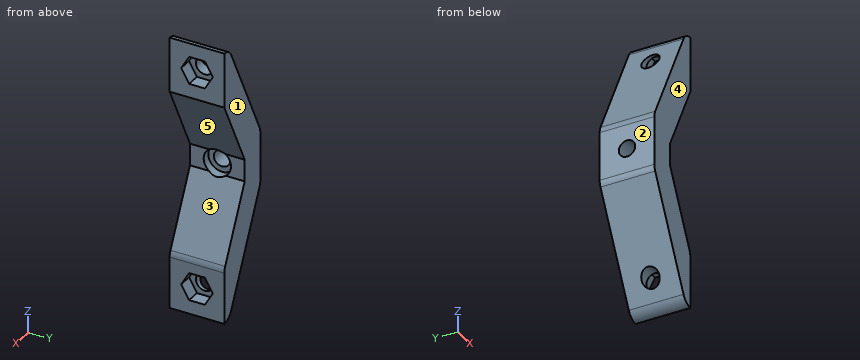
Autodesk Inventor part; units mm, degrees
ref_plane "YZ Plane" through (0, 0, 0) normal (1, 0, 0) x (0, 1, 0)
ref_plane "XZ Plane" through (0, 0, 0) normal (0, 1, 0) x (-1, 0, 0)
ref_plane "XY Plane" through (0, 0, 0) normal (0, 0, 1) x (1, 0, 0)
sketch "Sketch1" plane through (0, 0, 0) normal (0, 1, 0) x (-1, 0, 0)
  line L0 (0, 0) -> (-20, 0)
  line L1 (-20, 0) -> (-20, -40)
  line L2 (-20, -40) -> (0, 0)
  line L3 (-21.5, -50) -> (-18.5, -50)
  line L4 (-18.5, -50) -> (-18.5, -30)
  line L5 (-18.5, -30) -> (-21.5, -30)
  line L6 (-21.5, -30) -> (-21.5, -50)
  line L7 (-21.5, -50) -> (-18.5, -30) construction
  line L8 (-18.5, -50) -> (-21.5, -30) construction
  line L9 (1.5, 10) -> (-1.5, 10)
  line L10 (-1.5, 10) -> (-1.5, -10)
  line L11 (-1.5, -10) -> (1.5, -10)
  line L12 (1.5, -10) -> (1.5, 10)
  line L13 (1.5, 10) -> (-1.5, -10) construction
  line L14 (-1.5, 10) -> (1.5, -10) construction
  line L15 (-1.5, 10) -> (-21.5, -30)
  line L16 (1.5, -10) -> (-18.5, -50)
  line L17 (1.5, -10) -> (1.5, 10)
  line L18 (1.5, -10) -> (1.5, 10)
  line L19 (1.5, 10) -> (-8.5, 10)
  line L20 (-8.5, 10) -> (-8.5, -10)
  line L21 (-8.5, -10) -> (1.5, -10)
  line L22 (1.5, -10) -> (1.5, 10)
  line L23 (0, 0) -> (10, 0)
  line L24 (0, 0) -> (10, 0) construction
  line L25 (-20, 40) -> (0, 0)
  line L26 (-21.5, 50) -> (-18.5, 50)
  line L27 (-18.5, 50) -> (-18.5, 30)
  line L28 (-18.5, 30) -> (-21.5, 30)
  line L29 (-21.5, 30) -> (-21.5, 50)
  line L30 (-1.5, -10) -> (-1.5, 10)
  line L31 (-1.5, 10) -> (1.5, 10)
  line L32 (-1.5, -10) -> (-21.5, 30)
  line L33 (1.5, 10) -> (-18.5, 50)
  line L34 (1.5, 10) -> (1.5, -10)
  point P0 (-7.3579, -1.7157)
  point P1 (-11.5, -10)
  point P2 (-11.5, -10)
  point P3 (-8.5, -4)
  point P4 (-8.5, 4)
  dimension "d0" = 20
  dimension "d1" = 40
  dimension "d2" = 3
  dimension "d3" = 20
  dimension "d4" = 3
  dimension "d5" = 20
  dimension "d31" = 10
  dimension "d32" = 20
  dimension "d42" = 10
  dimension "d43" = 0
extrude "Extrusion1" add sketch "Sketch1" along normal blind 20 contours L2 L10 L0 | L23 L12 L11 L10 L2 | L25 L10 L9 L12 L23 | L0 L10 L25 | L10 L2 L32 L0 | L0 L15 L25 L10 | L10 L32 L2 | L25 L15 L10 | L15 L20 L0 | L32 L20 L19 L25 L15 | L32 L2 L21 L20 L15 | L0 L20 L32 | L32 L21 L2 | L11 L16 L4 L2 L21 | L9 L19 L25 L27 L33 | L15 L25 L19 | L20 L21 L2 L4 L5 L1 L15 | L32 L28 L27 L25 L19 L20 | L3 L6 L5 L1 L2 L4 | L27 L28 L29 L26 | L1 L5 L15 | L2 L1 L5 L4
sketch "Sketch2" plane through (-1.5, 0, -10) normal (-1, 0, 0) x (0, 0, 1)
  circle A0 centre (10, 10) radius 3
  line L0 (0, 0) -> (20, 0)
  line L1 (20, 0) -> (20, 20)
  point P0 (10, 0)
  dimension "d8" = 6
  dimension "d9" = 10
  dimension "d44" = 10
sketch "Sketch3" plane through (21.5, 0, -30) normal (1, 0, 0) x (0, 0, -1)
  circle A0 centre (10, 10) radius 3.25
  line L0 (0, 20) -> (20, 20)
  line L1 (20, 0) -> (20, 20)
  point P0 (-30, 0)
  dimension "d11" = 6.5
  dimension "d12" = 10
  dimension "d13" = 10
extrude "Extrusion2" cut sketch "Sketch2" against normal through all
extrude "Extrusion3" cut sketch "Sketch3" against normal through all
sketch "Sketch4" plane through (21.5, 0, -30) normal (1, 0, 0) x (0, 0, -1)
  circle A0 centre (10, 10) radius 3.25
  line L0 (10, 15.7735) -> (15, 12.8868)
  line L1 (15, 12.8868) -> (15, 7.1132)
  line L2 (15, 7.1132) -> (10, 4.2265)
  line L3 (10, 4.2265) -> (5, 7.1132)
  line L4 (5, 7.1132) -> (5, 12.8868)
  line L5 (5, 12.8868) -> (10, 15.7735)
  line L6 (20, 0) -> (20, 20)
  point P0 (-30, 0)
  point P1 (10, 10)
  dimension "d19" = 10
extrude "Extrusion4" cut sketch "Sketch4" against normal blind 5
fillet "Fillet2" radius 5 1 edges at (21.5, 10, -30)
mirror "Mirror1" about plane through (0, 0, 0) normal (0, 0, 1) of "Extrusion4", "Extrusion3"
sketch "Sketch7" plane through (8.5, 0, 4) normal (1, 0, 0) x (0, 0, -1)
  circle A0 centre (4, 10) radius 3
  circle A1 centre (4, 10) radius 5
  point P0 (4, 0)
  dimension "d52" = 10
extrude "Extrusion6" cut sketch "Sketch7" along normal mid plane 6 contours A0 | A1
fillet "Fillet8" radius 5 2 edges at (-1.5, 10, 10) (-1.5, 10, -10)
fillet "Fillet9" radius 5 2 edges at (18.5, 10, 50) (18.5, 10, -50)
ref_plane "Work Plane1" through (0, 0, 0) normal (0, 0, 1) x (1, 0, 0)
properties part number "Bottom_Foot_Standoff" material "PET Plastic"
For this review, take the finished solid that the model builds, in its own axes (mm). Face numbers are marked on the shaded views. A direction names the side the tool comes from. Round coordinates to 2 decimals unless told otherwise and drop trailing zeros. Loops run counter-clockwise (first coordinate to the right, second up) from the corner with the lowest first, then second, coordinate; pieces in that order, holes last. Notation, with made-up numbers: (-15, -8.5) - (34, -8.5) arc R13 ccw to (34, 6.5) - close; hole circle Ø6 at (15, 45.5). An arc over 180 degrees is marked (long way). Use one line per item in the form item = value.
Item 1: For line 1 (Y direction, x = 6.6, z = 0); line 2 (Y direction, x = 1.75, z = 0); line 3 (Z direction, x = 15.5, y = 10), list the stretches that pass through material, from the lowest coordinate up.
Answers:
line_1 = 0 to 5, 15 to 20
line_2 = 0 to 7, 13 to 20
line_3 = -44 to -43.25, -36.75 to -18, 18 to 36.75, 43.25 to 44
Item 2: Clearance check with flat-ended pins moving along their axes: P1, Ø4, axis at x = 1, z = 22.5, coming from the -Y side; P2, Ø3.5, axis at y = 16, z = -1.5, coming from the +X side; P3, Ø2.5, axis at x = 19, y = 9.5, coming from the +Z side; P4, Ø3, axis at x = 15, y = 9, coming from the -Z side. State where each tip first meets the part, or that it passes through.
Answers:
P1 = through
P2 = 8.5
P3 = 49.82
P4 = -46
Item 3: Consider section A-A on z = 0. Write out the cut boundary in (x, y), then the cut area to 3 significant figures.
Answers:
outline = (-1.5, 0) - (8.5, 0) - (8.5, 5) - (5.5, 5) - (5.5, 7) - (-1.5, 7) - close; (-1.5, 13) - (5.5, 13) - (5.5, 15) - (8.5, 15) - (8.5, 20) - (-1.5, 20) - close
area = 128 mm^2
Item 4: Mouldability with a two-part tool opening along X and no side actions: class the marked faces 1, 2 and 3 as +X half, -X half, draft (parallel to the pull), parting line (faces both ways), or undercut.
Answers:
face_1 = draft
face_2 = -X half
face_3 = +X half
Item 5: Tool access review of the marked faces 4 and 5: name each direction out of +Z, -Z, +X, -X, +Y, -Y from which nothing blocks a thin tool from reaching the whole face with its end or side.
Answers:
face_4 = +Z, -Z, +X, -X, -Y
face_5 = +X, +Y, -Y
Item 6: Consider section C-C on y = 2. Write out the cut boundary in (x, z), then the cut area to 3 significant figures.
Answers:
outline = (-1.5, -8.82) arc R5 ccw to (-0.97, -11.06) - (17.12, -47.24) arc R5 ccw to (21.5, -50) - (21.5, -31.18) arc R5 ccw to (20.97, -28.94) - (8.5, -4) - (8.5, 4) - (21.5, 30) - (21.5, 50) arc R5 ccw to (17.12, 47.24) - (-0.97, 11.06) arc R5 ccw to (-1.5, 8.82) - close
area = 1,050 mm^2
Item 7: Consider section D-D on x = 10.25. Write out the cut boundary in (y, z), then the cut area to 3 significant figures.
Answers:
outline = (0, -33.5) - (20, -33.5) - (20, -7.5) - (0, -7.5) - close; (0, 7.5) - (20, 7.5) - (20, 33.5) - (0, 33.5) - close
area = 1,040 mm^2
Item 8: Consider section B-B on x = 1. Write out the cut boundary in (y, z).
Answers:
outline = (0, -15) - (20, -15) - (20, 15) - (0, 15) - close; hole circle Ø6 at (10, 0)
